```python
from build123d import *

# Parameters (mm, degrees)
F0_R     = 18
F1_DEPTH = 4
F2_R     = 5
F3_D     = 6
F4_D     = 14.5


with BuildPart() as f1:
    # F0 (on Front) → F1 (new body)
    with BuildSketch(Plane.XZ):
        with BuildLine():
            Line((-12.5, 81.6506350946), (-12.5, 21.6506350946))
            ThreePointArc((-12.5, 21.6506350946), (-17.9406988245, -17.4106670087), (21.2661562924, -13.1434621219))
            ThreePointArc((21.2661562924, -13.1434621219), (24.242434448, 6.1077305141), (12.5, 21.6506350946))
            Line((12.5, 21.6506350946), (12.5, 49.7071421427))
            Line((12.5, 49.7071421427), (12.5, 81.6506350946))
            Line((12.5, 81.6506350946), (-12.5, 81.6506350946))
        make_face()
        Circle(F0_R, mode=Mode.SUBTRACT)
        with BuildLine():
            ThreePointArc((12.5, 21.6506350946), (24.242434448, 6.1077305141), (21.2661562924, -13.1434621219))
            Line((21.2661562924, -13.1434621219), (46.9090475237, 28.3468033545))
            ThreePointArc((46.9090475237, 28.3468033545), (22.7720659342, 28.8896918508), (35, 49.7071421427))
            Line((35, 49.7071421427), (12.5, 49.7071421427))
            Line((12.5, 49.7071421427), (12.5, 21.6506350946))
        make_face()
        with BuildLine():
            ThreePointArc((35, 49.7071421427), (22.7720659342, 28.8896918508), (46.9090475237, 28.3468033545))
            ThreePointArc((46.9090475237, 28.3468033545), (48.4671204296, 31.8813523767), (49, 35.7071421427))
            ThreePointArc((49, 35.7071421427), (44.8994949366, 45.6066370793), (35, 49.7071421427))
        make_face()
    extrude(amount=F1_DEPTH)

    # F2
    f2_edges = [f1.edges().sort_by_distance(p)[0] for p in [
        (12.5, -2, 81.650635),
        (12.5, -2, 49.707142),
        (21.266156, -2, -13.143462),
        (-12.5, -2, 21.650635),
        (-12.5, -2, 81.650635),
    ]]
    fillet(f2_edges, radius=F2_R)

    # F3 (through all)
    with Locations(Plane(origin=(0, 0, 0), x_dir=(1, 0, 0), z_dir=(0, 1, 0))):
        with Locations((0, -31.6506350946), (0, -71.6506350946)):
            Hole(F3_D / 2)

    # F4 (through all)
    with Locations(Plane(origin=(0, 0, 0), x_dir=(1, 0, 0), z_dir=(0, 1, 0))):
        with Locations((35, -35.7071421427)):
            Hole(F4_D / 2)


solid = f1.part
```
Here's how the part is built. I have some questions about the finished solid (model axes, mm). A direction names the side the tool comes from. Coordinates: 2 decimals unless noted, no trailing zeros. Write each loop counter-clockwise with the first axis right and the second up, starting at its lowest first coordinate (ties: lowest second). Pieces come first, ordered by that corner, then holes. Notation, with made-up numbers: M -3,0 L 18,0 A23 cw 18,33 Z; hole C 86,68.25 d4. An arc over 180 degrees is marked long. Answer as CSV lines item,"result". Start each with the question number.
Q1. Suppose I cut it at B-B, the plane z = -2.5. List the corners of the cut face in (x, y) for me, then the cut area to 3 significant figures.
Q2. Suppose I cut it at A-A, the plane x = 0. List the corners of the cut face in (y, z) for me, then the cut area to 3 significant figures.
Q3. If we mould it in two halves opening along X, with no side actions, what happens to faces 4 (the cylindrical face through (42.243, -2.028, 35.388)), 5 (the cylindrical face through (0.391, -2.028, 28.676)), 6 (the flat face through (0, -2, 81.651)), 7 (the cylindrical face through (11.07, -2.03, 80.15))? For each: pulls with the +X half, pulls with the -X half, needs draft (parallel to the pull), parting line crosses it, or undercut.
Q4. Suppose I cut it at D-D, the plane y = -2. List the corners of the cut face in (x, z) for me, then the cut area to 3 significant figures.
Q5. I need wall thicknesses on probe 1 along Z at (x, y) = (0, -1.1); probe 2 along X at (y, z) = (-2.25, 31.5); probe 3 along X at (y, z) = (-0.6, 61). Which ranges of each line are inside material? Lowest first, please. Write a range as [from, to].
Q6. Will these pins go through, and if not, where does the flat tip stop? pin 1 Ø5.5 at (x, z) = (0, 31.65) entering from +Y; pin 2 Ø5 at (x, z) = (-10, 43) entering from +Y; pin 3 Ø2 at (x, y) = (28, -1) entering from +Z; pin 4 Ø2 at (y, z) = (-2.5, 39) entering from -X.
Q7. For faces 1 (the flat face through (-12.5, -2, 51)), 2 (the flat face through (11, 0, 29)), 3 (the flat face through (12.5, -2, 66)), which set-ups out of +Z, -Z, +X, -X, +Y, -Y let a thin tool reach every point of the face, with its end or its side?
Q8. Suppose I cut it at C-C, the plane x = 41. List the corners of the cut face in (y, z) for me.
Entries:
1,outline,"M -24.87,-4 L -17.83,-4 L -17.83,0 L -24.87,0 Z; M 17.83,-4 L 27.84,-4 L 27.84,0 L 17.83,0 Z"
1,area,"68.3 mm²"
2,outline,"M -4,-25 L 0,-25 L 0,-18 L -4,-18 Z; M -4,18 L 0,18 L 0,28.65 L -4,28.65 Z; M -4,34.65 L 0,34.65 L 0,68.65 L -4,68.65 Z; M -4,74.65 L 0,74.65 L 0,81.65 L -4,81.65 Z"
2,area,"235 mm²"
3,face 4,"undercut"
3,face 5,"undercut"
3,face 6,"needs draft"
3,face 7,"pulls with the +X half"
4,outline,"M -14.58,20.31 A25 ccw long 21.27,-13.14 L 46.91,28.35 A14 ccw 35,49.71 L 17.5,49.71 A5 cw 12.5,54.71 L 12.5,76.65 A5 ccw 7.5,81.65 L -7.5,81.65 A5 ccw -12.5,76.65 L -12.5,24.37 A5 cw Z; hole C 0,0 d36; hole C 0,31.65 d6; hole C 0,71.65 d6; hole C 35,35.71 d14.5"
4,area,"3,450 mm²"
5,probe 1,"z = [-25, -18], [18, 28.65], [34.65, 68.65], [74.65, 81.65]"
5,probe 2,"x = [-12.5, -3], [3, 29.1], [40.9, 48.35]"
5,probe 3,"x = [-12.5, 12.5]"
6,pin 1,"passes through"
6,pin 2,"stops at y = 0"
6,pin 3,"stops at z = 49.71"
6,pin 4,"stops at x = -12.5"
7,face 1,"+Z, -X, +Y, -Y"
7,face 2,"+Z, -Z, +X, -X, +Y"
7,face 3,"+Z, +X, +Y, -Y"
8,outline,"M -4,18.79 L 0,18.79 L 0,31.64 L -4,31.64 Z; M -4,39.78 L 0,39.78 L 0,48.36 L -4,48.36 Z"
